Could you check a few things on this drawing? It's one solid part, dimensions in mm from its lowest x, y, z. A direction names the side the tool comes from. Give positions to 0.01 mm unless a question says otherwise; leave off trailing zeros. Order: outer loops, then holes, each group sorted by start corner. A loop starts at its lowest first (then second) coordinate and runs counter-clockwise, first axis right, second up. Notation, with made-up numbers: (65, 72) -> (96, 72) arc R16 ccw to (96, 97) -> close; hole circle Ø4 at (73, -11.5). An arc over 180 degrees is marked (long way). Write each question's results on one line, items separated by ' | '.
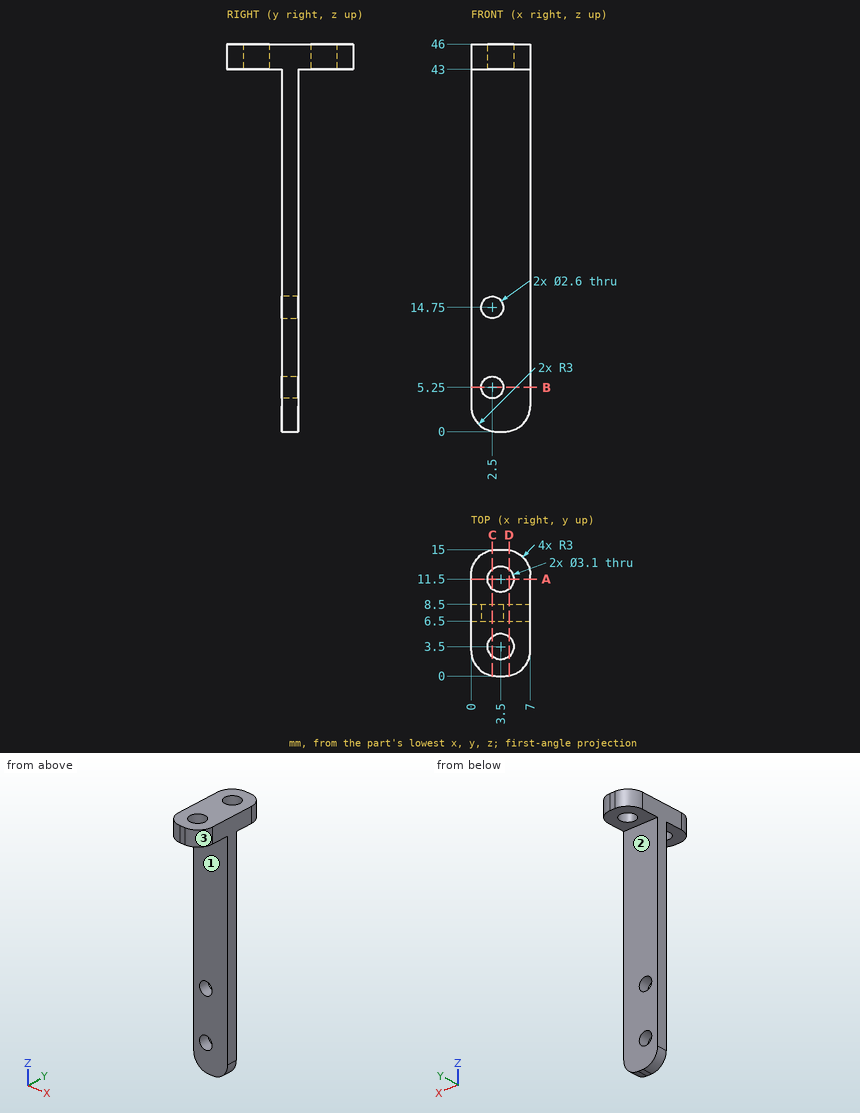
Q1. I need wall thicknesses on line 1 along X through (y, z) = (7.75, 5.25); line 2 along Y through (x, z) = (6, 37); line 3 along Z through (x, y) = (1, 5.5). Which ranges of each line are inside material? Lowest first, please.
Here are the results:
line 1: x = 0 to 1.2, 3.8 to 7 | line 2: y = 6.5 to 8.5 | line 3: z = 43 to 46
Q2. Suppose I cut it at C-C on x = 2.5. Please give me the cut outline in (y, z).
Here are the results:
outline: (0.04, 43) -> (2.32, 43) -> (2.32, 46) -> (0.04, 46) -> close; (4.68, 43) -> (6.5, 43) -> (6.5, 16.05) -> (8.5, 16.05) -> (8.5, 43) -> (10.32, 43) -> (10.32, 46) -> (4.68, 46) -> close; (6.5, 0.04) -> (8.5, 0.04) -> (8.5, 3.95) -> (6.5, 3.95) -> close; (6.5, 6.55) -> (8.5, 6.55) -> (8.5, 13.45) -> (6.5, 13.45) -> close; (12.68, 43) -> (14.96, 43) -> (14.96, 46) -> (12.68, 46) -> close
Q3. Suppose I cut it at D-D on x = 4.5. Please give me the cut outline in (y, z), and give its area (3 significant figures).
Here are the results:
outline: (0.04, 43) -> (2.32, 43) -> (2.32, 46) -> (0.04, 46) -> close; (4.68, 43) -> (6.5, 43) -> (6.5, 0.04) -> (8.5, 0.04) -> (8.5, 43) -> (10.32, 43) -> (10.32, 46) -> (4.68, 46) -> close; (12.68, 43) -> (14.96, 43) -> (14.96, 46) -> (12.68, 46) -> close | area: 116 mm²
Q4. For the marked faces 1, 2 and 3, which set-ups out of +Z, -Z, +X, -X, +Y, -Y let a thin tool reach every point of the face, with its end or its side?
Here are the results:
face 1: -Z, +X, -X, -Y | face 2: -Z, +X, -X, +Y | face 3: +Z, -Z, +X, -Y
Q5. Suppose I cut it at A-A on y = 11.5. Please give me the cut outline in (x, z).
Here are the results:
outline: (0, 43) -> (1.95, 43) -> (1.95, 46) -> (0, 46) -> close; (5.05, 43) -> (7, 43) -> (7, 46) -> (5.05, 46) -> close
Q6. I'm going to push flat-ended pins straight in: pin 1 Ø4 at (x, z) = (2.5, 5.25) entering from +Y; pin 2 Ø2 at (x, z) = (1, 15.5) entering from -Y. Where does each tip first touch, or does it pass through?
Here are the results:
pin 1: stops at y = 8.5 | pin 2: stops at y = 6.5
Q7. Suppose I cut it at B-B on z = 5.25. Please give me the cut outline in (x, y).
Here are the results:
outline: (0, 6.5) -> (1.2, 6.5) -> (1.2, 8.5) -> (0, 8.5) -> close; (3.8, 6.5) -> (7, 6.5) -> (7, 8.5) -> (3.8, 8.5) -> close
